Source: three-view drawing plus pictorial views. Frame: mm from the lowest corner of the part. A direction names the side the tool comes from. Round coordinates to 2 decimals unless told otherwise and drop trailing zeros. Order: outer loops, then holes, each group sorted by start corner. A loop starts at its lowest first (then second) coordinate and runs counter-clockwise, first axis right, second up. Notation, with made-up numbers: M -24,28.25 L -2,28.25 A26 cw -2,54.25 Z; hole C -20,22 d11. An arc over 180 degrees is marked long. Return JSON: item names as keys, results as strings. Group by question number.
Q1. Cut plane C-C on y = 19.5. Output: boundary loops of the cut face in (x, z).
Q2. Ray query, probe 1 along Y at (x, z) = (3.75, 12.5); probe 2 along Z at (x, y) = (1, 6); probe 3 along X at (y, z) = (19, 6.75). Return the intervals inside material, ascending.
Q3. Cut plane B-B on z = 7.7. Output: boundary loops of the cut face in (x, y), and give its area (3 significant figures).
Q4. Access query for the marked faces 1 and 2. Directions: +Z, -Z, +X, -X, +Y, -Y. A direction counts if a zero-diameter tool reaches every point of the face in a straight line with its end or side. Return the directions, or none.
Q5. Cut plane D-D on x = 10.25. Output: boundary loops of the cut face in (y, z), and give its area (4 significant figures).
Q6. Cut plane A-A on x = 7.7. Output: boundary loops of the cut face in (y, z).
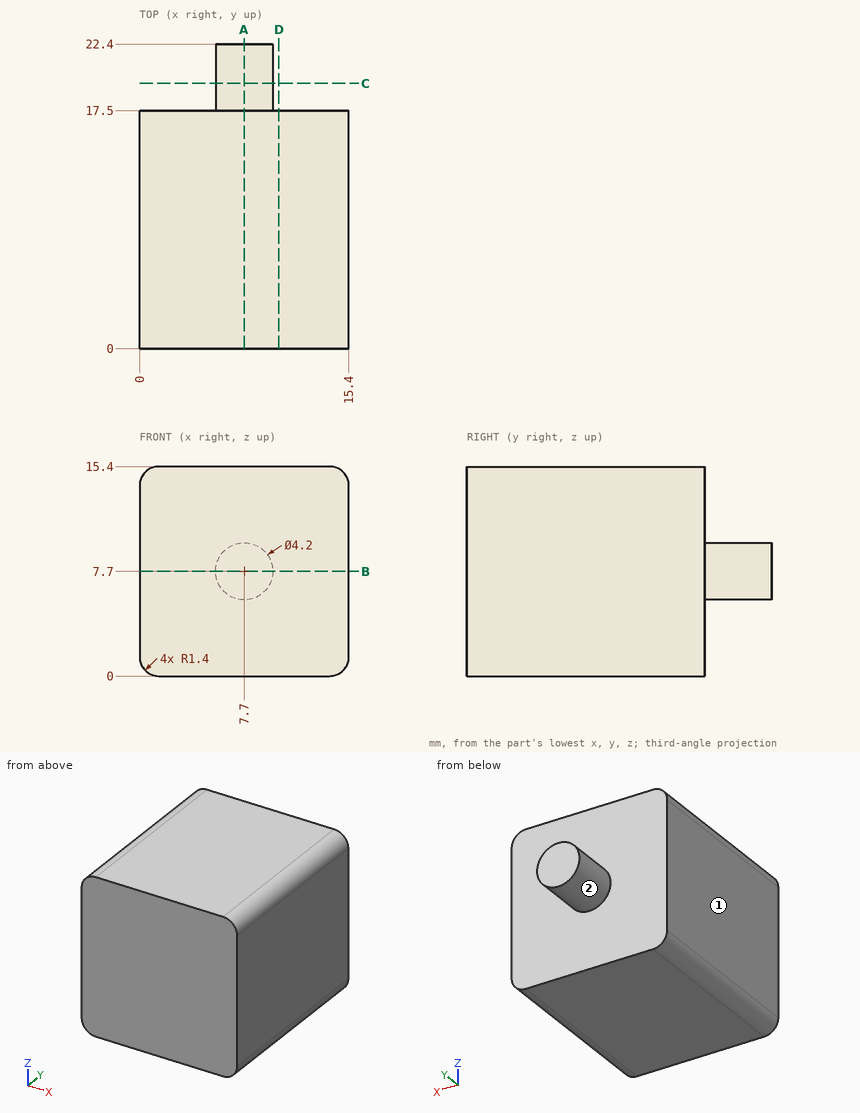
Result sheet:
{
 "1": {"outline": "C 7.7,7.7 d4.2"},
 "2": {"probe 1": "y = 0 to 17.5", "probe 2": "z = 0.06 to 15.34", "probe 3": "x = 5.83 to 9.57"},
 "3": {"outline": "M 0,0 L 15.4,0 L 15.4,17.5 L 9.8,17.5 L 9.8,22.4 L 5.6,22.4 L 5.6,17.5 L 0,17.5 Z", "area": "290 mm²"},
 "4": {"face 1": "+Z, -Z, -X, +Y, -Y", "face 2": "+Y"},
 "5": {"outline": "M 0,0 L 17.5,0 L 17.5,15.4 L 0,15.4 Z", "area": "269.5 mm²"},
 "6": {"outline": "M 0,0 L 17.5,0 L 17.5,5.6 L 22.4,5.6 L 22.4,9.8 L 17.5,9.8 L 17.5,15.4 L 0,15.4 Z"}
}
